```python
from build123d import *

# Parameters (mm, degrees)
SKETCH_1_R          = 1.65
EXTRUDE_1_DEPTH     = 3
CUT_EXTRUDE_1_DEPTH = 3
EXTRUDE_2_DEPTH     = 3
CUT_EXTRUDE_2_DEPTH = 3
FILLET_1_R          = 3
FILLET_2_R          = 3
SKETCH_7_R          = 1.65
CUT_EXTRUDE_4_DEPTH = 10
CUT_EXTRUDE_3_DEPTH = 3


with BuildPart() as part:
    # 草图1 → 凸台-拉伸1 (new body)
    with BuildSketch(Plane.XY):
        Polygon((-92.59237164, -12.480070197), (-72.241164341, -27), (-48.851597939, -10.5), (0, -10.5), (0, -0.5), (-50, -0.5), align=None)
        with Locations((-79.768579503, -13.030433694)):
            Circle(SKETCH_1_R, mode=Mode.SUBTRACT)
        with Locations((-70, -20)):
            Circle(SKETCH_1_R, mode=Mode.SUBTRACT)
    extrude(amount=EXTRUDE_1_DEPTH)

    # 镜向1: part across plane


with BuildPart() as part_1:
    add(part.part)
    add(part.part.mirror(Plane(origin=(0, -0.5, 3), x_dir=(0, 0, 1), z_dir=(-1, 0, 0))))

    # 草图2 → 切除-拉伸1 (cut)
    with BuildSketch(Plane.XY.offset(3)):
        Polygon((-92.59237164, -12.480070197), (-68.155479007, -24.11778291), (-72.241164341, -27), align=None)
        Polygon((92.59237164, -12.480070197), (68.155479007, -24.11778291), (72.241164341, -27), align=None)
    extrude(amount=-CUT_EXTRUDE_1_DEPTH, mode=Mode.SUBTRACT)

    # 草图3 → 凸台-拉伸2 (add)
    with BuildSketch(Plane.XY.offset(3)):
        Polygon((-25, -10.5), (-13, -33.83), (13, -33.83), (25, -10.5), align=None)
    extrude(amount=-EXTRUDE_2_DEPTH)

    # 草图4 → 切除-拉伸2 (cut)
    with BuildSketch(Plane.XY.offset(3)):
        Polygon((-11.661081625, -3.639004694), (-11.661081625, -0.5), (11.661081625, -0.5), (11.661081625, -3.639004694), (3.847453521, -18.83), (-3.847453521, -18.83), align=None)
    extrude(amount=-CUT_EXTRUDE_2_DEPTH, mode=Mode.SUBTRACT)

    # 圆角1
    fillet_1_edges = [part_1.edges().sort_by_distance(p)[0] for p in [
        (-48.851597939, -10.5, 1.5),
        (-92.59237164, -12.480070197, 1.5),
        (92.59237164, -12.480070197, 1.5),
        (48.851597939, -10.5, 1.5),
        (-68.155479007, -24.11778291, 1.5),
        (68.155479007, -24.11778291, 1.5),
        (-13, -33.83, 1.5),
        (13, -33.83, 1.5),
        (25, -10.5, 1.5),
        (-25, -10.5, 1.5),
        (11.661081625, -3.639004694, 1.5),
        (3.847453521, -18.83, 1.5),
        (-3.847453521, -18.83, 1.5),
        (-11.661081625, -3.639004694, 1.5),
    ]]
    fillet(fillet_1_edges, radius=FILLET_1_R)

    # 圆角2
    fillet_2_edges = [part_1.edges().sort_by_distance(p)[0] for p in [
        (11.661081625, -0.5, 1.5),
        (-11.661081625, -0.5, 1.5),
    ]]
    fillet(fillet_2_edges, radius=FILLET_2_R)

    # 草图7 → 切除-拉伸4 (cut)
    with BuildSketch(Plane.XY.offset(3)):
        with Locations((0, -30.53)):
            Circle(SKETCH_7_R)
    extrude(amount=-CUT_EXTRUDE_4_DEPTH, mode=Mode.SUBTRACT)

    # 草图5 → 切除-拉伸3 (cut)
    with BuildSketch(Plane.XY.offset(3)):
        with BuildLine():
            Line((-45, -3.9), (-25, -3.9))
            ThreePointArc((-25, -3.9), (-23.4, -5.5), (-25, -7.1))
            Line((-25, -7.1), (-45, -7.1))
            ThreePointArc((-45, -7.1), (-46.6, -5.5), (-45, -3.9))
        make_face()
        with BuildLine():
            Line((-67.050837469, -14.839231963), (-54.793781468, -6.192580693))
            ThreePointArc((-54.793781468, -6.192580693), (-52.564052692, -6.577690531), (-52.949162531, -8.807419307))
            Line((-52.949162531, -8.807419307), (-65.206218532, -17.454070576))
            ThreePointArc((-65.206218532, -17.454070576), (-67.435947308, -17.068960738), (-67.050837469, -14.839231963))
        make_face()
    cut_extrude_3 = extrude(amount=-CUT_EXTRUDE_3_DEPTH, mode=Mode.SUBTRACT)

    # 镜向2: 切除-拉伸3 across plane
    add(cut_extrude_3.mirror(Plane(origin=(0, 0, 0), x_dir=(0, 0, 1), z_dir=(1, 0, 0))), mode=Mode.SUBTRACT)


solid = part_1.part
```
Check sheet for the modelled part. Datum: model origin and axes. Units: mm. A direction names the side the tool comes from. Give positions to 0.01 mm unless a question says otherwise; leave off trailing zeros. Write each loop counter-clockwise with the first axis right and the second up, starting at its lowest first coordinate (ties: lowest second). Pieces come first, ordered by that corner, then holes.
Item 1: Draft check along Y on faces 6 (the face through (38, -10.5, 1)), 7 (the face through (-58.99, -13.07, 1.52)), 8 (the face through (-87.076, -12.9, 1.521)), 9 (the face through (23.4, -5.5, 1.5)). Enter one of: released by +Y, released by -Y, zero draft, split by the parting line, or undercut.
Item 2: Cross-section at D-D (x = 21). Enter the section's corners in (y, z).
Item 3: Cross-section at B-B (y = -30.53). Enter the section's corners in (x, z), and give its area (3 significant figures).
Item 4: Access from +Z, -Z, +X, -X, +Y, -Y to the whole of each face (thin tool, end or side, straight path). Record for faces 1 (the face through (3.6, -18.38, 1.48)), 2 (the face through (-33, -0.5, 1)), 3 (the face through (87.076, -12.9, 1.521)), 4 (the face through (18.928, -22.306, 1.521)), 5 (the face through (-35, -7.1, 2)).
Item 5: Cross-section at C-C (z = 0.5). Count the separate pieces of the cut face and the enclosed holes in it, and give its area (4 significant figures).
Item 6: Scan lines: L1, parallel to X at y = -15, z = 2.5; L2, parallel to Y at x = 0, z = 1.3; L3, parallel to X at y = -11, z = 1. Record each from-to range of solid material in increasing order.
Item 7: Gauge pin test, flat ends, axial feed: pin 1 (1.5 mm diameter, centred on x = -38.5, z = 2, fed in from -Y); pin 2 (1.5 mm diameter, centred on x = -59, z = 1.5, fed in from +Y); pin 3 (0.9 mm diameter, centred on x = 0, z = 2, fed in from +Y). Record the tip position at first contact, or that the pin passes through.
Item 8: Cross-section at A-A (x = 39.5). Enter the section's corners in (y, z).
Report:
1. face 6: released by -Y
1. face 7: undercut
1. face 8: split by the parting line
1. face 9: undercut
2. outline: (-18.28, 0) - (-0.5, 0) - (-0.5, 3) - (-18.28, 3) - close
3. outline: (-14.7, 0) - (-1.65, 0) - (-1.65, 3) - (-14.7, 3) - close; (1.65, 0) - (14.7, 0) - (14.7, 3) - (1.65, 3) - close
3. area: 78.3 mm2
4. face 1: +Z, -Z, +Y
4. face 2: +Z, -Z, +X, -X, +Y
4. face 3: +Z, -Z, +X
4. face 4: +Z, -Z, -Y
4. face 5: +Z, -Z
5. separate pieces: 1
5. enclosed holes: 9
5. area: 2,235 mm2
6. L1: x = -86.5 to -67.24, -61.73 to -55.23, -22.69 to -5.82, 5.82 to 22.69, 55.23 to 61.73, 67.24 to 86.5
6. L2: y = -33.83 to -32.18, -28.88 to -18.83
6. L3: x = -86.13 to -61.61, -56.06 to -49.56, -25.17 to -7.87, 7.87 to 25.17, 49.56 to 56.06, 61.61 to 86.13
7. pin 1: stops at y = -10.5
7. pin 2: stops at y = -2.82
7. pin 3: stops at y = -18.83
8. outline: (-10.5, 0) - (-7.1, 0) - (-7.1, 3) - (-10.5, 3) - close; (-3.9, 0) - (-0.5, 0) - (-0.5, 3) - (-3.9, 3) - close
